Build history of the part. All positions in model axes, mm. Round coordinates to 2 decimals unless told otherwise and drop trailing zeros. Loops run counter-clockwise (first coordinate to the right, second up) from the corner with the lowest first, then second, coordinate; pieces in that order, holes last. Notation, with made-up numbers: (66.5, 22) - (78.5, 22) arc R14 ccw to (78.5, 38) - close; hole circle Ø7 at (-36.75, 86). An arc over 180 degrees is marked (long way). Put each result on its own line as item: value. Start each with the question number.
from build123d import *

# Parameters (mm, degrees)
SKETCH_1_W      = 110
SKETCH_1_H      = 70
SKETCH_1_R      = 2.1
EXTRUDE_1_DEPTH = 3
FILLET_1_R      = 4


with BuildPart() as part:
    # 草图1 → 凸台-拉伸1 (new body)
    with BuildSketch(Plane.XY):
        Rectangle(SKETCH_1_W, SKETCH_1_H)
        with Locations((45, 20)):
            Circle(SKETCH_1_R, mode=Mode.SUBTRACT)
        with Locations((45, 0)):
            Circle(SKETCH_1_R, mode=Mode.SUBTRACT)
        with Locations((45, -20)):
            Circle(SKETCH_1_R, mode=Mode.SUBTRACT)
        with Locations(Location((-45, 20, 0), (0, 0, 180))):
            Circle(SKETCH_1_R, mode=Mode.SUBTRACT)
        with Locations(Location((-45, 0, 0), (0, 0, 180))):
            Circle(SKETCH_1_R, mode=Mode.SUBTRACT)
        with Locations(Location((-45, -20, 0), (0, 0, 180))):
            Circle(SKETCH_1_R, mode=Mode.SUBTRACT)
        with Locations((-7.5, 0)):
            Circle(SKETCH_1_R, mode=Mode.SUBTRACT)
        with Locations(Location((7.5, 0, 0), (0, 0, 180))):
            Circle(SKETCH_1_R, mode=Mode.SUBTRACT)
    extrude(amount=EXTRUDE_1_DEPTH)

    # 圆角1
    fillet_1_edges = [part.edges().sort_by_distance(p)[0] for p in [
        (55, -35, 1.5),
        (-55, -35, 1.5),
        (-55, 35, 1.5),
        (55, 35, 1.5),
    ]]
    fillet(fillet_1_edges, radius=FILLET_1_R)


solid = part.part
Item 1: Drill centre lines: probe 1 along Y at (x, z) = (-45, 2); probe 2 along Y at (x, z) = (7.5, 1.9); probe 3 along Y at (x, z) = (45.5, 2.1). Where is each one in solid material? Low to high. Write a range as [from, to].
Item 2: Drop a flat-ended pin along its axis: pin 1 Ø6.5 at (x, y) = (45, -20) entering from +Z. Give the stop position or say it passes through.
Item 3: Slice it at B-B (x = -7.5). Give the cut face in (y, z), plus the area to 3 significant figures.
Item 4: Slice it at D-D (x = 44). Give the cut face in (y, z), plus the area to 3 significant figures.
Item 5: Two-plate mould, pull along Y, no slides. Class faces 1 (the cylindrical face through (-9.6, 0.09, 1.48)), 2 (the cylindrical face through (46.13, -18.23, 1.48)), 3 (the cylindrical face through (-53.859, 33.797, 1.521)), 4 (the flat face through (-1, 0, 3)): pulls with the +Y half, pulls with the -Y half, needs draft (parallel to the pull), parting line crosses it, or undercut.
Item 6: Slice it at C-C (z = 2.4). Give the number of separate pieces and of enclosed holes in the cut face, plus the area to 3 significant figures.
Item 7: Slice it at A-A (y = 20). Give the cut face in (x, z).
Computed values:
1. probe 1: y = [-35, -22.1], [-17.9, -2.1], [2.1, 17.9], [22.1, 35]
1. probe 2: y = [-35, -2.1], [2.1, 35]
1. probe 3: y = [-35, -22.04], [-17.96, -2.04], [2.04, 17.96], [22.04, 35]
2. pin 1: stops at z = 3
3. outline: (-35, 0) - (-2.1, 0) - (-2.1, 3) - (-35, 3) - close; (2.1, 0) - (35, 0) - (35, 3) - (2.1, 3) - close
3. area: 197 mm^2
4. outline: (-35, 0) - (-21.85, 0) - (-21.85, 3) - (-35, 3) - close; (-18.15, 0) - (-1.85, 0) - (-1.85, 3) - (-18.15, 3) - close; (1.85, 0) - (18.15, 0) - (18.15, 3) - (1.85, 3) - close; (21.85, 0) - (35, 0) - (35, 3) - (21.85, 3) - close
4. area: 177 mm^2
5. face 1: undercut
5. face 2: undercut
5. face 3: pulls with the +Y half
5. face 4: needs draft
6. separate pieces: 1
6. enclosed holes: 8
6. area: 7,580 mm^2
7. outline: (-55, 0) - (-47.1, 0) - (-47.1, 3) - (-55, 3) - close; (-42.9, 0) - (42.9, 0) - (42.9, 3) - (-42.9, 3) - close; (47.1, 0) - (55, 0) - (55, 3) - (47.1, 3) - close
